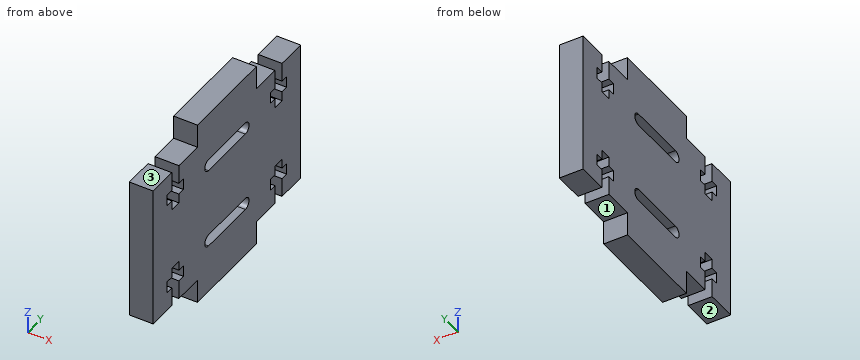
from build123d import *

# Parameters (mm, degrees)
BOSS_EXTRUDE1_DEPTH = 5
CUT_EXTRUDE1_DEPTH  = 6


with BuildPart() as part:
    # Sketch1 → Boss-Extrude1 (new body)
    with BuildSketch(Plane(origin=(0, 0, 0), x_dir=(0, 0, -1), z_dir=(1, 0, 0))):
        Polygon((-15, 50), (15, 50), (15, 35), (20, 35), (20, 15), (15, 15), (15, 0), (-15, 0), (-15, 15), (-20, 15), (-20, 35), (-15, 35), align=None)
        with BuildLine():
            Line((9.75, 31.25), (9.75, 18.75))
            ThreePointArc((9.75, 18.75), (8.5, 17.5), (7.25, 18.75))
            Line((7.25, 18.75), (7.25, 31.25))
            ThreePointArc((7.25, 31.25), (8.5, 32.5), (9.75, 31.25))
        make_face(mode=Mode.SUBTRACT)
        with BuildLine():
            Line((-9.75, 31.25), (-9.75, 18.75))
            ThreePointArc((-9.75, 18.75), (-8.5, 17.5), (-7.25, 18.75))
            Line((-7.25, 18.75), (-7.25, 31.25))
            ThreePointArc((-7.25, 31.25), (-8.5, 32.5), (-9.75, 31.25))
        make_face(mode=Mode.SUBTRACT)
    extrude(amount=BOSS_EXTRUDE1_DEPTH)

    # Sketch2 → Cut-Extrude1 (cut, through all)
    with BuildSketch(Plane(origin=(5, 0, 0), x_dir=(0, 0, -1), z_dir=(1, 0, 0))):
        Polygon((-15, 43.7), (-11, 43.7), (-11, 45.25), (-8.6, 45.25), (-8.6, 43.7), (-6.6, 43.7), (-6.6, 41.3), (-8.6, 41.3), (-8.6, 39.75), (-11, 39.75), (-11, 41.3), (-15, 41.3), align=None)
        Polygon((15, 41.3), (11, 41.3), (11, 39.75), (8.6, 39.75), (8.6, 41.3), (6.6, 41.3), (6.6, 43.7), (8.6, 43.7), (8.6, 45.25), (11, 45.25), (11, 43.7), (15, 43.7), align=None)
        Polygon((-15, 8.7), (-11, 8.7), (-11, 10.25), (-8.6, 10.25), (-8.6, 8.7), (-6.6, 8.7), (-6.6, 6.3), (-8.6, 6.3), (-8.6, 4.75), (-11, 4.75), (-11, 6.3), (-15, 6.3), align=None)
        Polygon((15, 6.3), (11, 6.3), (11, 4.75), (8.6, 4.75), (8.6, 6.3), (6.6, 6.3), (6.6, 8.7), (8.6, 8.7), (8.6, 10.25), (11, 10.25), (11, 8.7), (15, 8.7), align=None)
    extrude(amount=-CUT_EXTRUDE1_DEPTH, mode=Mode.SUBTRACT)


solid = part.part
CAD build for the part. Positions are in the model's coordinates, mm. Face numbers are marked on the shaded views. A direction names the side the tool comes from. Coordinates: 2 decimals unless noted, no trailing zeros. Write each loop counter-clockwise with the first axis right and the second up, starting at its lowest first coordinate (ties: lowest second). Pieces come first, ordered by that corner, then holes. Notation, with made-up numbers: M -16,52.25 L 11,52.25 A14 ccw 11,70.25 Z; hole C 42.5,65 d7. An arc over 180 degrees is marked long. Return JSON: item names as keys, results as strings.
Item 1: Which spindle directions (+Z, -Z, +X, -X, +Y, -Y) get a long thin tool onto all of the face, cutting with end or side? Do the marked faces 1, 2 and 3. Say none if no direction does.
Findings below:
{"face 1": "-Z, +X, -X, +Y", "face 2": "-Z, +X, -X, -Y", "face 3": "+Z, +X, -X, -Y"}
Item 2: Slice it at C-C, the plane y = 21. Write the cut outline in (x, z), and give its area (3 significant figures).
Findings below:
{"outline": "M 0,-20 L 5,-20 L 5,-9.75 L 0,-9.75 Z; M 0,-7.25 L 5,-7.25 L 5,7.25 L 0,7.25 Z; M 0,9.75 L 5,9.75 L 5,20 L 0,20 Z", "area": "175 mm2"}
Item 3: Slice it at B-B, the plane z = 8. Write the cut outline in (x, y), and give its area (3 significant figures).
Findings below:
{"outline": "M 0,0 L 5,0 L 5,6.3 L 0,6.3 Z; M 0,8.7 L 5,8.7 L 5,17.6 L 0,17.6 Z; M 0,32.4 L 5,32.4 L 5,41.3 L 0,41.3 Z; M 0,43.7 L 5,43.7 L 5,50 L 0,50 Z", "area": "152 mm2"}
Item 4: Drop flat-ended pins along their axis: pin 1 Ø1.2 at (x, z) = (1.5, 13.5) entering from -Y; pin 2 Ø0.5 at (x, y) = (3, 5.5) entering from -Z; pin 3 Ø1.7 at (x, y) = (2.5, 44.5) entering from +Z; pin 4 Ø1.5 at (x, z) = (2.5, 18) entering from -Y. Give the stop position or say it passes through.
Findings below:
{"pin 1": "stops at y = 0", "pin 2": "stops at z = -15", "pin 3": "stops at z = 15", "pin 4": "stops at y = 15"}
Item 5: Probe line 1 (Z direction, x = 3, y = 41); line 2 (Z direction, x = 2.3, y = 30.5); line 3 (Y direction, x = 2.6, z = -7). List the from-to ranges inside material, lowest first. Write a range as from..to.
Findings below:
{"line 1": "z = -15..-11, -8.6..8.6, 11..15", "line 2": "z = -20..-9.75, -7.25..7.25, 9.75..20", "line 3": "y = 0..6.3, 8.7..41.3, 43.7..50"}
Item 6: Slice it at D-D, the plane x = 2.65. State how many separate pieces and enclosed holes the cut face has, and give its area (3 significant figures).
Findings below:
{"separate pieces": "1", "enclosed holes": "2", "area": "1,520 mm2"}
Item 7: Slice it at A-A, the plane y = 40.5. Write the cut outline in (x, z).
Findings below:
{"outline": "M 0,-15 L 5,-15 L 5,-11 L 0,-11 Z; M 0,-8.6 L 5,-8.6 L 5,8.6 L 0,8.6 Z; M 0,11 L 5,11 L 5,15 L 0,15 Z"}
